For this review, take the finished solid that the model builds, in its own axes (mm). A direction names the side the tool comes from. Coordinates: 2 decimals unless noted, no trailing zeros. Write each loop counter-clockwise with the first axis right and the second up, starting at its lowest first coordinate (ties: lowest second). Pieces come first, ordered by that corner, then holes. Notation, with made-up numbers: (75.25, 10.5) -> (132.25, 10.5) arc R20 cw to (132.25, 49.5) -> close; hole circle Ø4 at (80.5, 65). An arc over 180 degrees is marked (long way). One line per item, written item: value. Start each with the question number.
1) Mouldability with a two-part tool opening along X and no side actions: class faces 4 (the cylindrical face through (-1, -74, 0)), 5 (the flat face through (-150, -74, 172)), 6 (the cylindrical face through (-21.68, -177.45, 202.38)) as released by +X, released by -X, zero draft, split by the parting line, or undercut.
2) Add section A-A (x = 0). State the section outline as (y, z) points.
3) Add section C-C (z = 59). State the section outline as (x, y) points.
4) Machinability: for faces 1 (the flat face through (4, -150, -56)), 2 (the cylindrical face through (-3.958, -248.6, -120.044)), 3 (the flat face through (152.147, -74, 296)), which of the approach directions +Z, -Z, +X, -X, +Y, -Y give a long, thin tool a straight path to every point of the face, cutting with its end or side? Answer none if there is none.
5) Add section B-B (y = -239). State the section outline as (x, z) points, and give its area (3 significant figures).
6) For pin 1 Ø1.5 at (x, y) = (54.5, -240.5) entering from +Z; pin 2 Ø1 at (x, y) = (50, -272.5) entering from +Z, all flat-tipped, find the tip position at first contact; note any pin that passes through.
7) Add section D-D (z = -178). State the section outline as (x, y) points, and give its area (3 significant figures).
8) For probe 1 along Z at (x, y) = (0, -253); probe 2 along Z at (x, y) = (0, -111); probe 3 along Y at (x, z) = (158, -166), list the stretches that pass through material, from the lowest coordinate up. Write a range as from..to.
from build123d import *

# Parameters (mm, degrees)
F2_DEPTH = 350
F3_DEPTH = 25
F4_R     = 100
F5_DEPTH = 350.001
F7_DEPTH = 150


with BuildPart() as f2:
    # F0 (on Front) → F2 (new body)
    with BuildSketch(Plane.XZ):
        with BuildLine():
            Line((300, -300), (300, 300))
            Line((300, 300), (-300, 300))
            Line((-300, 300), (-300, -300))
            Line((-300, -300), (-180, -300))
            ThreePointArc((-180, -300), (0, -120), (180, -300))
            Line((180, -300), (300, -300))
        make_face()
        with BuildLine():
            Line((-300, 300), (300, 300))
            ThreePointArc((300, 300), (0, 600), (-300, 300))
        make_face()
    extrude(amount=F2_DEPTH)

    # F1 (on face) → F3 (cut)
    with BuildSketch(Plane.XZ):
        with BuildLine():
            ThreePointArc((180, -300), (0, -120), (-180, -300))
            Line((-180, -300), (180, -300))
        make_face()
    extrude(amount=-F3_DEPTH, mode=Mode.SUBTRACT)

    # F4 (on face) → F5 (cut, through all)
    with BuildSketch(Plane.XZ.offset(350)):
        with Locations((0, 300)):
            Circle(F4_R)
    extrude(amount=-F5_DEPTH, mode=Mode.SUBTRACT)

    # F6 (on face) → F7 (cut)
    with BuildSketch(Plane(origin=(0, 0, 0), x_dir=(-1, 0, 0), z_dir=(0, 1, 0))):
        with BuildLine():
            ThreePointArc((150, 40.192379), (-1.242634, 0.002574), (-152.147139, 41.443917))
            Line((-152.147139, 41.443917), (-152.147139, 558.556083))
            ThreePointArc((-152.147139, 558.556083), (-260.426709, 448.922561), (-300, 300))
            Line((-300, 300), (-300, -300))
            Line((-300, -300), (-180, -300))
            ThreePointArc((-180, -300), (0, -120), (180, -300))
            Line((180, -300), (300, -300))
            Line((300, -300), (300, 300))
            ThreePointArc((300, 300), (260.876453, 448.133306), (153.710157, 557.629943))
            Line((153.710157, 557.629943), (150, 300))
            Line((150, 300), (150, 40.192379))
        make_face()
    extrude(amount=-F7_DEPTH, mode=Mode.SUBTRACT)


solid = f2.part
Numbers:
1. face 4: split by the parting line
1. face 5: released by -X
1. face 6: undercut
2. outline: (-350, -120) -> (-150, -120) -> (-150, 0) -> (0, 0) -> (0, 200) -> (-350, 200) -> close; (-350, 400) -> (0, 400) -> (0, 600) -> (-350, 600) -> close
3. outline: (-300, -350) -> (300, -350) -> (300, -150) -> (152.15, -150) -> (152.15, 0) -> (-150, 0) -> (-150, -150) -> (-300, -150) -> close
4. face 1: -Z, +Y
4. face 2: -Z, +Y, -Y
4. face 3: +Z, -Z, +X, +Y
5. outline: (-300, -300) -> (-180, -300) arc R180 cw to (180, -300) -> (300, -300) -> (300, 300) arc R300 ccw to (-300, 300) -> close; hole circle Ø200 at (0, 300)
5. area: 419,000 mm²
6. pin 1: z = 595.15
6. pin 2: z = 595.89
7. outline: (-300, -350) -> (-132.35, -350) -> (-132.35, -150) -> (-300, -150) -> close; (132.35, -350) -> (300, -350) -> (300, -150) -> (132.35, -150) -> close
7. area: 67,100 mm²
8. probe 1: -120..200, 400..600
8. probe 2: 0..200, 400..600
8. probe 3: -350..-150
